Design review of the part built by this model. Coordinates are the model's own, in mm. Give positions to 0.01 mm unless a question says otherwise; leave off trailing zeros. Order: outer loops, then holes, each group sorted by start corner. A loop starts at its lowest first (then second) coordinate and runs counter-clockwise, first axis right, second up. Notation, with made-up numbers: M 57,2 L 73,2 A11 ccw 73,14 Z; hole C 22,87 d9. An arc over 180 degrees is marked long. Answer as a JSON object with one key per item and string values.
from build123d import *

# Parameters (mm, degrees)
BOSS_EXTRUDE1_DEPTH = 3
CUT_EXTRUDE2_DEPTH  = 80
BOSS_EXTRUDE2_DEPTH = 3


with BuildPart() as part:
    # Sketch1 → Boss-Extrude1 (new body)
    with BuildSketch(Plane(origin=(40.618995436, 405.717520436, 71.391276418), x_dir=(0.935705749, -0.202672232, 0.288753733), z_dir=(-0.118950757, -0.951829224, -0.282616075))):
        Polygon((-9.093557887, 199.496352052), (122.645886532, 181.228380511), (87.83671653, -69.797887318), (-43.902727889, -51.529915777), align=None)
    extrude(amount=-BOSS_EXTRUDE1_DEPTH)

    # Sketch3 → Cut-Extrude2 (cut)
    with BuildSketch(Plane(origin=(184.762741438, 119.897305559, 240.069514855), x_dir=(0.516756682, 0.537673014, -0.66623589), z_dir=(0.567103814, 0.368008283, 0.736860345))):
        Polygon((970.937778761, -219.886702224), (970.937778761, 845.245168422), (-1124.286512281, 775.631358808), (-1124.286512281, -289.500511838), align=None)
    extrude(amount=CUT_EXTRUDE2_DEPTH, mode=Mode.SUBTRACT)

    # Sketch4 → Boss-Extrude2 (add)
    with BuildSketch(Plane(origin=(48.910383393, 391.374830059, 116.206579281), x_dir=(0.992857215, -0.11667261, -0.024940964), z_dir=(-0.118950757, -0.951829224, -0.282616075))):
        Polygon((83.713958284, -16.750212929), (96.993345394, -84.345811369), (209.443931521, -62.254508112), (207.834795901, -54.063581501), align=None)
    extrude(amount=-BOSS_EXTRUDE2_DEPTH)


solid = part.part
(1) We need section A-A (x = 66.5). Write out the cut boundary in (y, z).
Checked values:
{"outline": "M 361.15,210.6 L 417.8,19.8 L 420.72,20.59 L 364.85,208.75 Z"}
(2) Insertion check: pin 1 (10 mm diameter, centred on x = 55, z = 40, fed in from +Y); pin 2 (6 mm diameter, centred on x = 147, z = 90.5, fed in from +Y). Each pin has a flat end and moves straight along its axis. Give the tip position at first contact, or say it passes through.
Checked values:
{"pin 1": "stops at y = 418", "pin 2": "stops at y = 390.87"}
(3) We need section B-B (z = 132). Write out the cut boundary in (x, y).
Checked values:
{"outline": "M -8.87,393.91 L 124.99,377.18 L 125.52,380.26 L -8.33,396.99 Z"}
(4) To check wall thickness, follow L1, parallel to Y at x = 14.5, z = 246; L2, parallel to Y at x = 121, z = 73. State the ranges of each line that lie inside material, in increasing order. Write a range as from..to.
Checked values:
{"L1": "y = 357.14..360.29", "L2": "y = 395.19..398.35"}
